Check sheet for the drawn part. Datum: minimum x, y, z corner. Units: mm. Give positions to 0.01 mm unless a question says otherwise; leave off trailing zeros. Loops run counter-clockwise (first coordinate to the right, second up) from the corner with the lowest first, then second, coordinate; pieces in that order, holes last. Notation, with made-up numbers: (-21.75, 69) - (-15.75, 69) arc R13 cw to (-15.75, 89) - close; hole circle Ø3 at (0, 60). An arc over 180 degrees is marked (long way). Answer in a Markdown table with one row per item.
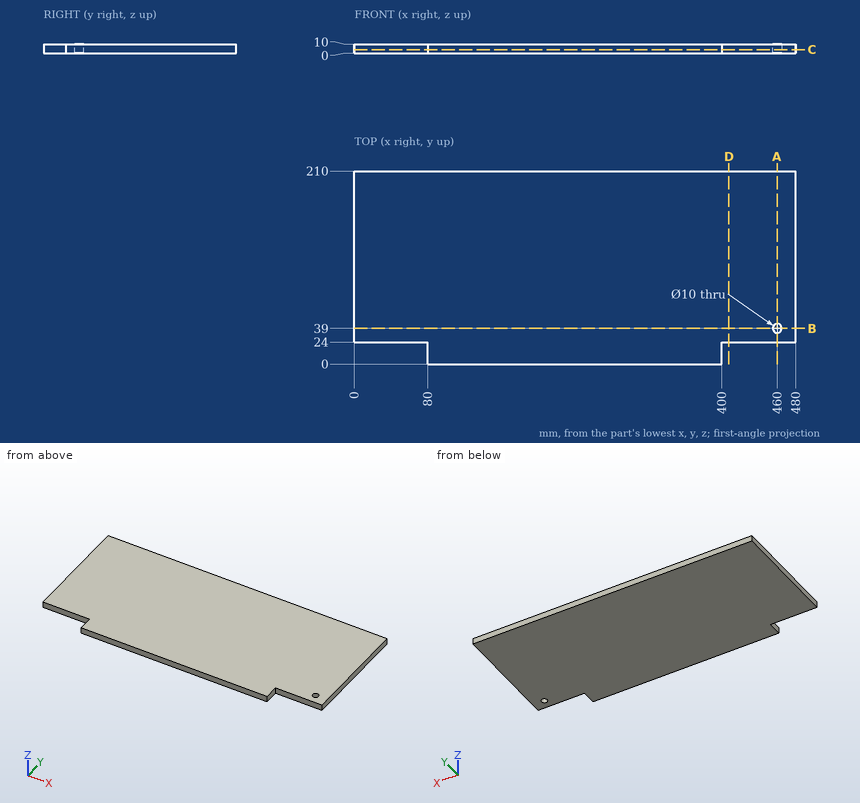
Q1. Sectioned sample at A-A (x = 460). Record the cut outline in (y, z).
Completed:
| item | result |
|---|---|
| outline | (24, 0) - (34, 0) - (34, 10) - (24, 10) - close; (44, 0) - (210, 0) - (210, 10) - (44, 10) - close |
Q2. Sectioned sample at D-D (x = 407.5). Record the cut outline in (y, z).
Completed:
| item | result |
|---|---|
| outline | (24, 0) - (210, 0) - (210, 10) - (24, 10) - close |
Q3. Sectioned sample at C-C (z = 4). Record the cut outline in (x, y).
Completed:
| item | result |
|---|---|
| outline | (0, 24) - (80, 24) - (80, 0) - (400, 0) - (400, 24) - (480, 24) - (480, 210) - (0, 210) - close; hole circle Ø10 at (460, 39) |
Q4. Go/stop test with a flat-tipped pin: P1, Ø11.5, axis at x = 460, y = 39, coming from the +Z side. Record where the tip stops, or that it passes through.
Completed:
| item | result |
|---|---|
| P1 | z = 10 |
Q5. Thickness scan on line 1 (Y direction, x = 460, z = 5.5); line 2 (Y direction, x = 427, z = 8.25); line 3 (X direction, y = 11, z = 0.5). Record the ranges inside material, lowest first.
Completed:
| item | result |
|---|---|
| line 1 | 24 to 34, 44 to 210 |
| line 2 | 24 to 210 |
| line 3 | 80 to 400 |
Q6. Sectioned sample at B-B (y = 39). Record the cut outline in (x, z), and give its area (3 significant figures).
Completed:
| item | result |
|---|---|
| outline | (0, 0) - (455, 0) - (455, 10) - (0, 10) - close; (465, 0) - (480, 0) - (480, 10) - (465, 10) - close |
| area | 4,700 mm^2 |
